from build123d import *

# Parameters (mm, degrees)
SKETCH1_W           = 24.13
SKETCH1_H           = 24.13
BOSS_EXTRUDE1_DEPTH = 5.08
SKETCH2_R           = 3.302
CUT_EXTRUDE1_DEPTH  = 1.27
SKETCH3_R           = 3.175
BOSS_EXTRUDE2_DEPTH = 1.27


with BuildPart() as part:
    # Sketch1 → Boss-Extrude1 (new body)
    with BuildSketch(Plane(origin=(0, 0, 0), x_dir=(1, 0, 0), z_dir=(0, 1, 0))):
        Rectangle(SKETCH1_W, SKETCH1_H)
    extrude(amount=BOSS_EXTRUDE1_DEPTH)

    # Sketch2 → Cut-Extrude1 (cut)
    with BuildSketch(Plane(origin=(0, 0, 0), x_dir=(1, 0, 0), z_dir=(0, 1, 0))):
        with Locations(Location((0, 0, 0), (0, 0, 270))):
            Circle(SKETCH2_R)
    extrude(amount=CUT_EXTRUDE1_DEPTH, mode=Mode.SUBTRACT)

    # Sketch3 → Boss-Extrude2 (add)
    with BuildSketch(Plane(origin=(0, 5.08, 0), x_dir=(1, 0, 0), z_dir=(0, 1, 0))):
        with Locations(Location((0, 0, 0), (0, 0, 90))):
            Circle(SKETCH3_R)
    extrude(amount=BOSS_EXTRUDE2_DEPTH)


solid = part.part
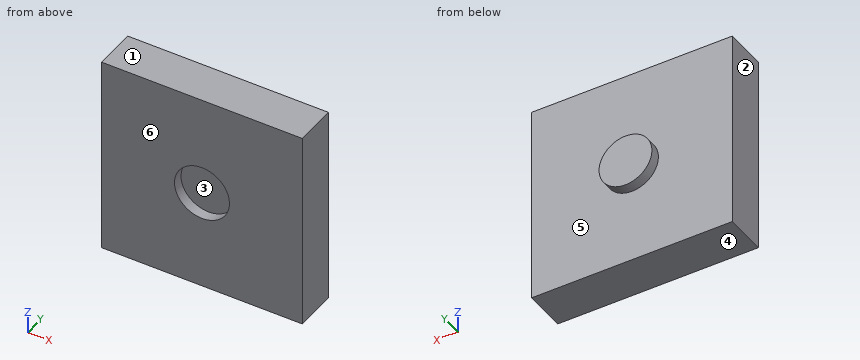
Could you check a few things on this model? Use its own coordinates, in mm. Face numbers are marked on the shaded views. A direction names the side the tool comes from. Give positions to 0.01 mm unless a question says otherwise; leave off trailing zeros. Order: outer loops, then holes, each group sorted by start corner. A loop starts at its lowest first (then second) coordinate and runs counter-clockwise, first axis right, second up. Notation, with made-up numbers: (-24, 18) - (30, 18) arc R16 cw to (30, 27) - close; hole circle Ø3 at (-21.75, 63.25). An arc over 180 degrees is marked (long way). Return JSON: item names as keys, results as strings. Group by question number.
Q1. Which directions (+Z, -Z, +X, -X, +Y, -Y) give clear straight access to the entire face, cutting with the end or side of a thin tool? Please do the marked faces 5 and 6.
Q2. Thinking about a two-plate mould opening in Z: for the marked faces 1, 2, 3 and 4, which applies, pulls with the +Z half, pulls with the -Z half, needs draft (parallel to the pull), parting line crosses it, or undercut?
Q3. Suppose I cut it at C-C, the plane y = 0.5. Please give me the cut outline in (x, z) (3 decimals), and give its area (3 significant figures).
Q4. Please list where these lines run through material, in increasing order: line 1 along X through (y, z) = (0.9, 0) (3 decimals); line 2 along Y through (x, z) = (9.5, -3.5); line 3 along Y through (x, z) = (0.5, -3). Write a range as [from, to].
Q5. Suppose I cut it at A-A, the plane x = 0. Please give me the cut outline in (y, z) (3 decimals).
Q6. Will this pin go through, and if not, where does the flat tip stop? pin 1 Ø3 at (x, z) = (-1, -9.5) entering from +Y.
Q7. Suppose I cut it at D-D, the plane y = 6. Please give me the cut outline in (x, z) (3 decimals).
Q8. Suppose I cut it at B-B, the plane z = 0. Please give me the cut outline in (x, y) (3 decimals).
Resolved:
{
 "1": {"face 5": "+Y", "face 6": "+Z, -Z, +X, -X, -Y"},
 "2": {"face 1": "pulls with the +Z half", "face 2": "needs draft", "face 3": "undercut", "face 4": "pulls with the -Z half"},
 "3": {"outline": "(-12.065, -12.065) - (12.065, -12.065) - (12.065, 12.065) - (-12.065, 12.065) - close; hole circle Ø6.604 at (0, 0)", "area": "548 mm2"},
 "4": {"line 1": "x = [-12.065, -3.302], [3.302, 12.065]", "line 2": "y = [0, 5.08]", "line 3": "y = [1.27, 6.35]"},
 "5": {"outline": "(0, -12.065) - (5.08, -12.065) - (5.08, -3.175) - (6.35, -3.175) - (6.35, 3.175) - (5.08, 3.175) - (5.08, 12.065) - (0, 12.065) - (0, 3.302) - (1.27, 3.302) - (1.27, -3.302) - (0, -3.302) - close"},
 "6": {"pin 1": "stops at y = 5.08"},
 "7": {"outline": "circle Ø6.35 at (0, 0)"},
 "8": {"outline": "(-12.065, 0) - (-3.302, 0) - (-3.302, 1.27) - (3.302, 1.27) - (3.302, 0) - (12.065, 0) - (12.065, 5.08) - (3.175, 5.08) - (3.175, 6.35) - (-3.175, 6.35) - (-3.175, 5.08) - (-12.065, 5.08) - close"}
}
